Autodesk Fusion 360 part; units mm, degrees
sketch "スケッチ1" plane through (0, 0, 0) normal (0, 0, 1) x (1, 0, 0)
  line L0 (-9.5, 140) -> (-80.5, 140)
  line L1 (-80.5, 140) -> (-80.5, -140)
  line L2 (-80.5, -140) -> (-9.5, -140)
  line L3 (80.5, -30) -> (80.5, 130)
  line L4 (74.75, 130) -> (-80.5, -140) construction
  line L5 (-9.5, 140) -> (-9.5, 130)
  line L6 (-9.5, 130) -> (80.5, 130)
  line L7 (-80.5, -140) -> (-9.5, -140) construction
  line L8 (80.5, -50) -> (-9.5, -140)
  line L9 (80.5, -50) -> (-9.5, -50)
  line L10 (-9.5, -50) -> (-9.5, -30)
  line L11 (-9.5, -30) -> (80.5, -30)
  line L12 (-80.5, 140) -> (17.25, -30) construction
  line L13 (28.75, -50) -> (47.6429, -82.8571) construction
  dimension "d2" = 280
  dimension "d5" = 71
  dimension "d7" = 90
  dimension "d8" = 20
extrude "押し出し1" add sketch "スケッチ1" along normal blind 6
chamfer "面取り1" distance 25 angle 45 2 edges at (-80.5, -140, 3) (-80.5, 140, 3)
sketch "スケッチ2" plane through (0, 0, 6) normal (0, 0, 1) x (-1, 0, 0)
  line L0 (55.5, -140) -> (80.5, -115)
  line L1 (80.5, -115) -> (80.5, 115)
  line L2 (80.5, 115) -> (55.5, 140)
  line L3 (55.5, 140) -> (9.5, 140)
  line L4 (9.5, 140) -> (-80.5, 50)
  line L5 (-80.5, 50) -> (9.5, 50)
  line L6 (9.5, 50) -> (9.5, 30)
  line L7 (9.5, 30) -> (-80.5, 30)
  line L8 (-80.5, 30) -> (-80.5, -130)
  line L9 (-80.5, -130) -> (9.5, -130)
  line L10 (9.5, -130) -> (9.5, -140)
  line L11 (9.5, -140) -> (55.5, -140)
  line L12 (-80.5, -130) -> (-40.5, -130) construction
  line L13 (-40.5, -130) -> (-40.5, -80) construction
  line L14 (-40.5, -80) -> (-80.5, -80) construction
  line L15 (-80.5, -80) -> (-80.5, -130) construction
  line L16 (-40.5, -80) -> (-40.5, -20) construction
  point P0 (-40.5, -80)
  point P1 (-40.5, -20)
  dimension "d12" = 40
  dimension "d13" = 50
  dimension "d14" = 60
hole "穴1" at (40.5, 80, 6) at (40.5, 20, 6) direction (0, 0, -1) diameter 18 end through all
equation "d5 = 25 mm + 46 mm"
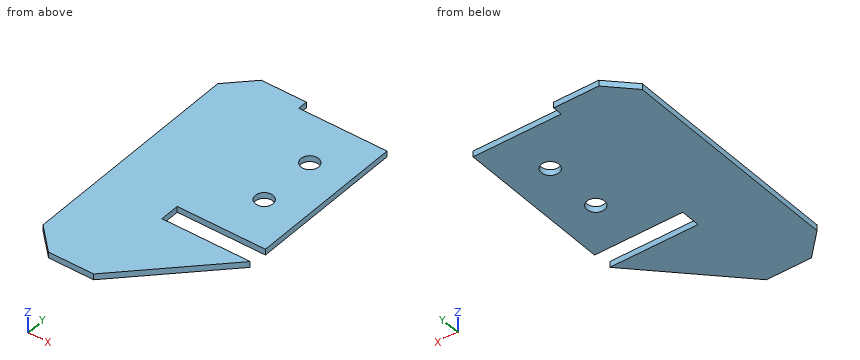
Could you check a few things on this model? Use its own coordinates, in mm. Coordinates: 2 decimals unless noted, no trailing zeros. Loops run counter-clockwise (first coordinate to the right, second up) from the corner with the lowest first, then second, coordinate; pieces in that order, holes last.
1) Imagine slicing it at D-D (y = 80). List the corners of the cut face in (x, z) for me, and give its area (3 significant figures).
Reported:
outline: (-80.5, 0) - (31.5, 0) - (31.5, 6) - (-80.5, 6) - close; (49.5, 0) - (80.5, 0) - (80.5, 6) - (49.5, 6) - close
area: 858 mm2
2) Imagine slicing it at B-B (x = 40.5). List the corners of the cut face in (y, z) for me.
Reported:
outline: (-90, 0) - (-50, 0) - (-50, 6) - (-90, 6) - close; (-30, 0) - (11, 0) - (11, 6) - (-30, 6) - close; (29, 0) - (71, 0) - (71, 6) - (29, 6) - close; (89, 0) - (130, 0) - (130, 6) - (89, 6) - close
3) Will these pins go through, and if not, where does the flat tip stop? pin 1 Ø1.8 at (x, z) = (44, 3) entering from +Y; pin 2 Ø20.5 at (x, y) = (40.5, 20) entering from -Z; pin 3 Ø1.8 at (x, z) = (29, 4.5) entering from -Y.
Reported:
pin 1: stops at y = 130
pin 2: stops at z = 0
pin 3: stops at y = -102.4
4) Please list where these lines run through material, in increasing order: line 1 along Y through (x, z) = (40.5, 4.05); line 2 along X through (y, z) = (79, 4.2); line 3 along X through (y, z) = (20, 4.6).
Reported:
line 1: y = -90 to -50, -30 to 11, 29 to 71, 89 to 130
line 2: x = -80.5 to 31.56, 49.44 to 80.5
line 3: x = -80.5 to 31.5, 49.5 to 80.5
5) Imagine slicing it at C-C (z = 4.05). List the corners of the cut face in (x, y) for me.
Reported:
outline: (-80.5, -115) - (-55.5, -140) - (-9.5, -140) - (80.5, -50) - (-9.5, -50) - (-9.5, -30) - (80.5, -30) - (80.5, 130) - (-9.5, 130) - (-9.5, 140) - (-55.5, 140) - (-80.5, 115) - close; hole circle Ø18 at (40.5, 20); hole circle Ø18 at (40.5, 80)
6) Imagine slicing it at A-A (x = 18). List the corners of the cut face in (y, z) for me.
Reported:
outline: (-112.5, 0) - (-50, 0) - (-50, 6) - (-112.5, 6) - close; (-30, 0) - (130, 0) - (130, 6) - (-30, 6) - close
